Work out the finished part from the listing and answer in its coordinate system (mm). A direction names the side the tool comes from. Round coordinates to 2 decimals unless told otherwise and drop trailing zeros. Loops run counter-clockwise (first coordinate to the right, second up) from the corner with the lowest first, then second, coordinate; pieces in that order, holes last. Notation, with made-up numbers: (-14, 44.5) - (38, 44.5) arc R15 cw to (38, 65.5) - close; hole circle Ø7 at (30, -40). An arc over 180 degrees is marked (long way). Return JSON: item names as keys, results as strings.
from build123d import *

# Parameters (mm, degrees)
BOSS_EXTRUDE1_DEPTH            = 10
SKETCH2_W                      = 1.9
SKETCH2_H                      = 0.9
CUT_EXTRUDE1_DEPTH             = 12.703418304
SKETCH3_W                      = 1.9
SKETCH3_H                      = 0.9
CUT_EXTRUDE2_DEPTH             = 12.703418304
CUT_EXTRUDE3_DEPTH             = 12.703418304
F_4_2_4_2_DIAMETER_HOLE1_D     = 4.2
F_4_2_4_2_DIAMETER_HOLE1_DEPTH = 4.5
FILLET1_R                      = 0.2


with BuildPart() as part:
    # Sketch1 → Boss-Extrude1 (new body)
    with BuildSketch(Plane.XY.offset(5)):
        Polygon((4.9, -1), (4.9, 0.9), (-4.9, 0.9), (-4.9, -1), (-2.3, -3.6), (2.3, -3.6), align=None)
    extrude(amount=-BOSS_EXTRUDE1_DEPTH)

    # Sketch2 → Cut-Extrude1 (cut, through all)
    with BuildSketch(Plane(origin=(0, 0, -5), x_dir=(-1, 0, 0), z_dir=(0, 0, -1))):
        with Locations((3.95, 0.45)):
            Rectangle(SKETCH2_W, SKETCH2_H)
    extrude(amount=-CUT_EXTRUDE1_DEPTH, mode=Mode.SUBTRACT)

    # Sketch3 → Cut-Extrude2 (cut, through all)
    with BuildSketch(Plane(origin=(0, 0, -5), x_dir=(-1, 0, 0), z_dir=(0, 0, -1))):
        with Locations((-3.95, 0.45)):
            Rectangle(SKETCH3_W, SKETCH3_H)
    extrude(amount=-CUT_EXTRUDE2_DEPTH, mode=Mode.SUBTRACT)

    # Sketch4 → Cut-Extrude3 (cut, through all)
    with BuildSketch(Plane(origin=(0, 0, -5), x_dir=(-1, 0, 0), z_dir=(0, 0, -1))):
        Polygon((0.4, 0.9), (-0.4, 0.9), (0, 0.5), align=None)
    extrude(amount=-CUT_EXTRUDE3_DEPTH, mode=Mode.SUBTRACT)

    # Ø4.2 (4.2) Diameter Hole1
    with Locations(Plane(origin=(0, -3.6, 0), x_dir=(-1, 0, 0), z_dir=(0, -1, 0))):
        with Locations((0, 0)):
            Hole(F_4_2_4_2_DIAMETER_HOLE1_D / 2, depth=F_4_2_4_2_DIAMETER_HOLE1_DEPTH)

    # Fillet1
    fillet1_edges = [part.edges().sort_by_distance(p)[0] for p in [
        (4.9, 0, 0),
        (3, 0, 0),
        (-4.9, -1, 0),
        (3, 0.9, 0),
        (-3, 0, 0),
        (0.4, 0.9, -3.530776406),
        (0, 0.5, 3.55),
        (-0.4, 0.9, -3.530776406),
        (4.9, -1, 0),
        (-3, 0.9, 0),
        (0, 0.5, -3.55),
        (-0.4, 0.9, 3.530776406),
        (-4.9, 0, 0),
        (-2.3, -3.6, 0),
        (0.4, 0.9, 3.530776406),
        (2.3, -3.6, 0),
    ]]
    fillet(fillet1_edges, radius=FILLET1_R)


solid = part.part
1) Flat-ended cylindrical pins translate along their axes: pin 1 (1.2 mm diameter, centred on x = -4.5, z = 2, fed in from +Y); pin 2 (2 mm diameter, centred on y = -2.5, z = 3, fed in from -X); pin 3 (2 mm diameter, centred on x = 3.5, z = 4, fed in from -Y). Find the tip coordinate at first contact, or state that the pin passes through.
Verdict:
{"pin 1": "stops at y = 0", "pin 2": "stops at x = -4.4", "pin 3": "stops at y = -3.4"}
2) A tool of negligible diameter and unlimited length cuts with its end or side. For faces 1 (the flat face through (-4, 0, 0)), 2 (the flat face through (4, 0, 0)), 3 (the flat face through (-2.4, 0.9, 0.1)), from which of +Z, -Z, +X, -X, +Y, -Y can it reach the whole face along a straight path? Write none if from no direction.
Verdict:
{"face 1": "+Z, -Z, -X, +Y", "face 2": "+Z, -Z, +X, +Y", "face 3": "+Z, -Z, +X, -X, +Y"}
3) Section A-A (z = 0) is taken. Give the vertices of the cut face in (x, y).
Verdict:
{"outline": "(-4.9, -0.92) arc R0.2 ccw to (-4.84, -1.06) - (-2.36, -3.54) arc R0.2 ccw to (-2.22, -3.6) - (-2.1, -3.6) - (-2.1, 0.9) - (-2.8, 0.9) arc R0.2 ccw to (-3, 0.7) - (-3, 0.2) arc R0.2 cw to (-3.2, 0) - (-4.7, 0) arc R0.2 ccw to (-4.9, -0.2) - close; (2.1, -3.6) - (2.22, -3.6) arc R0.2 ccw to (2.36, -3.54) - (4.84, -1.06) arc R0.2 ccw to (4.9, -0.92) - (4.9, -0.2) arc R0.2 ccw to (4.7, 0) - (3.2, 0) arc R0.2 cw to (3, 0.2) - (3, 0.7) arc R0.2 ccw to (2.8, 0.9) - (2.1, 0.9) - close"}
4) Section C-C (y = -2.7) is taken. Give the vertices of the cut face in (x, z), and give its area (3 significant figures).
Verdict:
{"outline": "(-3.2, -5) - (3.2, -5) - (3.2, 5) - (-3.2, 5) - close; hole circle Ø4.2 at (0, 0)", "area": "50.1 mm2"}
5) Section B-B (x = 0) is taken. Give the vertices of the cut face in (y, z).
Verdict:
{"outline": "(-3.6, -5) - (0.58, -5) - (0.58, -2.1) - (-3.6, -2.1) - close; (-3.6, 2.1) - (0.58, 2.1) - (0.58, 5) - (-3.6, 5) - close"}
6) Determine the mould class of faces 4 (the flat face through (0, -1, -5)), 5 (the cylindrical face through (2.003, -1.319, -0.631)), 6 (the flat face through (0, -3.6, 2.3)) for opening direction Z: pulls with the +Z half, pulls with the -Z half, needs draft (parallel to the pull), parting line crosses it, or undercut.
Verdict:
{"face 4": "pulls with the -Z half", "face 5": "undercut", "face 6": "needs draft"}
7) Section D-D (z = 4.25) is taken. Give the vertices of the cut face in (x, y).
Verdict:
{"outline": "(-4.9, -0.92) arc R0.2 ccw to (-4.84, -1.06) - (-2.36, -3.54) arc R0.2 ccw to (-2.22, -3.6) - (2.22, -3.6) arc R0.2 ccw to (2.36, -3.54) - (4.84, -1.06) arc R0.2 ccw to (4.9, -0.92) - (4.9, -0.2) arc R0.2 ccw to (4.7, 0) - (3.2, 0) arc R0.2 cw to (3, 0.2) - (3, 0.7) arc R0.2 ccw to (2.8, 0.9) - (0.48, 0.9) arc R0.2 ccw to (0.34, 0.84) - (0.14, 0.64) arc R0.2 cw to (-0.14, 0.64) - (-0.34, 0.84) arc R0.2 ccw to (-0.48, 0.9) - (-2.8, 0.9) arc R0.2 ccw to (-3, 0.7) - (-3, 0.2) arc R0.2 cw to (-3.2, 0) - (-4.7, 0) arc R0.2 ccw to (-4.9, -0.2) - close"}
8) Find the intervals of material crossed by L1, parallel to Z at x = 0, y = -2.6; L2, parallel to X at y = -2.2, z = -0.25; L3, parallel to Z at x = -1.75, y = 0.1, in increasing order.
Verdict:
{"L1": "z = -5 to -2.1, 2.1 to 5", "L2": "x = -3.7 to -2.09, 2.09 to 3.7", "L3": "z = -5 to -1.16, 1.16 to 5"}
